Can you work these out from the model? Positions are in its coordinate system, mm. Face numbers are marked on the shaded views. A direction names the side the tool comes from. Give positions to 0.01 mm unless a question says otherwise; leave off trailing zeros. Loops run counter-clockwise (first coordinate to the right, second up) from the corner with the lowest first, then second, coordinate; pieces in that order, holes last. Notation, with made-up numbers: (46, -6.75) - (75, -6.75) arc R19 cw to (75, 26.25) - close; hole circle Ø2 at (49.5, 47.5). An arc over 180 degrees is marked (long way). Answer as a JSON object with one key per item and string values. Group by question number.
Item 1: Which directions (+Z, -Z, +X, -X, +Y, -Y) give clear straight access to the entire face, cutting with the end or side of a thin tool? Please do the marked faces 1, 2, 3 and 4.
Item 2: Suppose I cut it at B-B on z = 18. Write out the boundary of the cut face in (x, y).
Item 3: Thinking about a two-plate mould opening in Z: for the marked faces 5, 6, 7 and 8, which applies, pulls with the +Z half, pulls with the -Z half, needs draft (parallel to the pull), parting line crosses it, or undercut?
Item 4: Suppose I cut it at C-C on y = -7.5. Write out the boundary of the cut face in (x, z), and give its area (3 significant figures).
Item 5: Please list where these lines run through material, in increasing order: L1, parallel to Y at x = 32.5, z = 5.25; L2, parallel to X at y = 22, z = -2; L3, parallel to Y at x = -48, z = 0.25.
Item 6: Will these pins go through, and if not, where does the flat tip stop? pin 1 (5 mm diameter, centred on x = -31.5, z = -3.5, fed in from +Y); pin 2 (3 mm diameter, centred on x = -44.5, z = 2.5, fed in from -Y); pin 3 (3 mm diameter, centred on x = 15, y = -26.5, fed in from +Z).
Item 7: Suppose I cut it at A-A on x = 7. Write out the boundary of the cut face in (y, z).
Item 8: Suppose I cut it at D-D on y = 26.5. Write out the boundary of the cut face in (x, z), and give its area (3 significant figures).
Autodesk Fusion 360 part; units mm, degrees
sketch "Sketch1" plane through (0, 0, 0) normal (0, 0, 1) x (1, 0, 0)
  circle A0 centre (-48, 0) radius 6
  line L0 (-48, -17) -> (0, -17)
  line L1 (-48, 17) -> (0, 17)
  line L2 (0, 17) -> (0, -17)
  arc A1 (-48, 17) -> (-48, -17) centre (-48, 0) ccw
  dimension "d1" = 48
  dimension "d2" = 12
  dimension "d3" = 34
  dimension "d5" = 48
extrude "Extrude1" add sketch "Sketch1" along normal mid plane 16
sketch "Sketch2" plane through (0, 0, 0) normal (0, 1, 0) x (1, 0, 0)
  line L0 (0, 8) -> (65, 8)
  line L1 (0, 8) -> (0, -45)
  line L2 (0, -45) -> (12, -45)
  line L3 (12, -45) -> (12, -9)
  line L4 (12, -9) -> (53, -9)
  line L5 (65, 8) -> (65, -45)
  line L6 (65, -45) -> (53, -45)
  line L7 (53, -45) -> (53, -9)
  dimension "d8" = 65
  dimension "d9" = 53
  dimension "d10" = 12
  dimension "d11" = 41
  dimension "d12" = 53
  dimension "d13" = 12
extrude "Extrude2" add sketch "Sketch2" along normal mid plane 76
fillet "Fillet1" radius 16 4 edges at (6, 38, 45) (6, -38, 45) (59, -38, 45) (59, 38, 45)
sketch "Sketch3" plane through (0, 0, 0) normal (-1, 0, 0) x (0, -1, 0)
  arc A0 (38, 29) -> (22, 45) centre (22, 29) ccw
  line L0 (22, 45) -> (-22, 45)
  arc A1 (-22, 45) -> (-38, 29) centre (-22, 29) ccw
  line L1 (-38, 29) -> (-38, -8)
  line L2 (-38, -8) -> (-17, -8)
  line L3 (-17, -8) -> (-17, 8)
  line L4 (-17, 8) -> (17, 8)
  line L5 (17, 8) -> (17, -8)
  line L6 (17, -8) -> (38, -8)
  line L7 (38, -8) -> (38, 29)
  line L8 (-22, 23) -> (22, 23)
  arc A2 (22, 23) -> (22, 35) centre (22, 29) ccw
  line L9 (22, 35) -> (-22, 35)
  arc A3 (-22, 35) -> (-22, 23) centre (-22, 29) ccw
  line L10 (-22, 29) -> (22, 29) construction
  dimension "d18" = 44
  dimension "d19" = 6
  dimension "d21" = 21
extrude "Extrude3" cut sketch "Sketch3" against normal blind 65 contours L8 A2 L9 A3
sketch "Sketch4" plane through (0, 0, 9) normal (0, 0, 1) x (-1, 0, 0)
  line L0 (-53, 38) -> (-53, -38)
  line L1 (-53, -38) -> (-12, -38)
  line L2 (-12, -38) -> (-12, 38)
  line L3 (-12, 38) -> (-53, 38)
  point P0 (-32.5, -22)
  point P1 (-32.5, 22)
  dimension "d24" = 44
  dimension "d25" = 16
  dimension "d26" = 20.5
hole "Hole1" at (32.5, 22, 9) at (32.5, -22, 9) direction (0, 0, -1) diameter 12 depth 65 tip angle 118
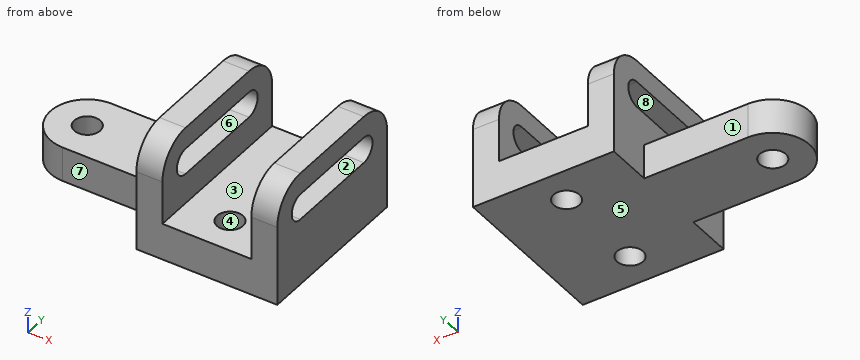
Worked out:
{
 "1": {"face 1": "+Z, -Z, -X, +Y", "face 2": "+X, -X", "face 3": "+Z, +Y, -Y", "face 4": "+Z, -Z"},
 "2": {"outline": "(0, -38) - (12, -38) - (12, 38) - (0, 38) - close; (53, -38) - (65, -38) - (65, 38) - (53, 38) - close"},
 "3": {"face 5": "pulls with the -Z half", "face 6": "undercut", "face 7": "needs draft", "face 8": "undercut"},
 "4": {"outline": "(-63.26, -8) - (65, -8) - (65, 23) - (53, 23) - (53, 9) - (12, 9) - (12, 23) - (0, 23) - (0, 8) - (-63.26, 8) - close; (0, 35) - (12, 35) - (12, 45) - (0, 45) - close; (53, 35) - (65, 35) - (65, 45) - (53, 45) - close", "area": "2,690 mm2"},
 "5": {"L1": "y = -38 to -28, -16 to 16, 28 to 38", "L2": "x = 0 to 26.5, 38.5 to 65", "L3": "y = -17 to -6, 6 to 17"},
 "6": {"pin 1": "stops at y = 17", "pin 2": "stops at y = -17", "pin 3": "stops at z = 9"},
 "7": {"outline": "(-38, -8) - (38, -8) - (38, 29) arc R16 ccw to (22, 45) - (-22, 45) arc R16 ccw to (-38, 29) - close; hole (-22, 23) - (22, 23) arc R6 ccw to (22, 35) - (-22, 35) arc R6 ccw to start"},
 "8": {"outline": "(0, -8) - (28.53, -8) - (28.53, 9) - (12, 9) - (12, 25.03) - (0, 25.03) - close; (0, 32.97) - (12, 32.97) - (12, 44.35) - (0, 44.35) - close; (36.47, -8) - (65, -8) - (65, 25.03) - (53, 25.03) - (53, 9) - (36.47, 9) - close; (53, 32.97) - (65, 32.97) - (65, 44.35) - (53, 44.35) - close", "area": "1,630 mm2"}
}
